Check sheet for the modelled part. Datum: model origin and axes. Units: mm. Give positions to 0.01 mm unless a question says otherwise; leave off trailing zeros. Order: outer loops, then holes, each group sorted by start corner. A loop starts at its lowest first (then second) coordinate and runs counter-clockwise, first axis right, second up. Notation, with made-up numbers: (25, 52) -> (82, 52) arc R23 cw to (82, 73) -> close; hole circle Ø4 at (43, 77). An arc over 180 degrees is marked (long way). Answer in a Markdown table with one row per item. Add a question column.
(1) Release check for a two-part mould opening along Y. For faces 1 (the face through (0, -6, 15)), 2 (the face through (-0.867, -3.905, 7.605)), 3 (the face through (33.384, 10.513, 7.416)) record: released by +Y, released by -Y, zero draft, split by the parting line, or undercut.
(2) Cross-section at A-A (z = 12.25). Record the cut outline in (x, y).
(3) Thickness scan on L1, parallel to Z at x = 28, y = 7.5; L2, parallel to X at y = -23.5, z = 12; L3, parallel to X at y = 31.5, z = 10.5. Record the ranges inside material, lowest first. Write a range as [from, to].
(4) Go/stop test with flat-tipped pins: pin 1 (6 mm diameter, centred on x = 26.5, y = -17, fed in from +Z); pin 2 (5 mm diameter, centred on y = 3.5, z = 11, fed in from +X); pin 3 (1 mm diameter, centred on x = -8, y = 28, fed in from -Z). Record where each tip stops, or that it passes through.
```python
from build123d import *

# Parameters (mm, degrees)
SKETCH_2_R          = 35
EXTRUDE_1_DEPTH     = 15
SKETCH_5_R          = 4
CUT_EXTRUDE_1_DEPTH = 20


with BuildPart() as part:
    # 스케치2 → 보스-돌출1 (new body)
    with BuildSketch(Plane.XY):
        Circle(SKETCH_2_R)
    extrude(amount=EXTRUDE_1_DEPTH)

    # 스케치5 → 컷-돌출1 (cut)
    with BuildSketch(Plane.XY.offset(15)):
        Circle(SKETCH_5_R)
    extrude(amount=-CUT_EXTRUDE_1_DEPTH, mode=Mode.SUBTRACT)

    # 컷-스윕2: sweep along a curve in space
    with BuildLine() as sweep_2_path:
        ThreePointArc((35, 0, 0), (24.748737342, 24.748737342, 0), (0, 35, 0))
        ThreePointArc((0, 35, 0), (-24.748737342, 24.748737342, 0), (-35, 0, 0))
        ThreePointArc((-35, 0, 0), (-24.748737342, -24.748737342, 0), (0, -35, 0))
        ThreePointArc((0, -35, 0), (24.748737342, -24.748737342, 0), (35, 0, 0))
    # 스케치4 → 컷-스윕2 (sweep, cut)
    with BuildSketch(Plane(origin=(0, 0, 0), x_dir=(1, 0, 0), z_dir=(0, 1, 0))):
        Polygon((-35, -1.5), (-26.493077271, 0), (-35, 0), align=None)
        Polygon((-35, -15), (-26.493077271, -15), (-35, -13.5), align=None)
    sweep(path=sweep_2_path.line, mode=Mode.SUBTRACT)


solid = part.part
```
Answer below:
| question | item | result |
|---|---|---|
| 1 | face 1 | zero draft |
| 1 | face 2 | undercut |
| 1 | face 3 | split by the parting line |
| 2 | outline | circle Ø70 at (0, 0); hole circle Ø8 at (0, 0) |
| 3 | L1 | z = [0.44, 14.56] |
| 3 | L2 | x = [-25.94, 25.94] |
| 3 | L3 | x = [-15.26, 15.26] |
| 4 | pin 1 | stops at z = 14.65 |
| 4 | pin 2 | stops at x = 34.99 |
| 4 | pin 3 | stops at z = 0.38 |
